from build123d import *

# Parameters (mm, degrees)
F0_W      = 200
F0_H      = 100
F0_W_2    = 196
F0_H_2    = 96
F1_DEPTH  = 40
F2_DEPTH  = 2
F3_W      = 62
F3_H      = 96
F4_DEPTH  = 25
F5_W      = 60
F5_H      = 96
F6_DEPTH  = 25
F8_DEPTH  = 25
F9_W      = 14
F9_H      = 10
F10_DEPTH = 5
F12_W     = 10
F12_H     = 10
F13_DEPTH = 5
F14_R     = 2
F15_W     = 20
F15_H     = 15
F16_DEPTH = 2
F17_W     = 15
F17_H     = 10
F18_DEPTH = 2
F19_W     = 86
F19_H     = 2
F20_DEPTH = 25
F21_W     = 25
F21_H     = 15
F22_DEPTH = 88
F23_W     = 40
F23_H     = 30
F24_DEPTH = 2
F25_W     = 20
F25_H     = 15
F26_DEPTH = 2


with BuildPart() as f1:
    # F0 (on Front) → F1 (new body)
    with BuildSketch(Plane.XZ):
        with Locations((-23.666499, -18.106852)):
            Rectangle(F0_W, F0_H)
        with Locations((-23.666499, -18.106852)):
            Rectangle(F0_W_2, F0_H_2, mode=Mode.SUBTRACT)
    extrude(amount=F1_DEPTH)

    # F0 (on Front) → F2 (join)
    with BuildSketch(Plane.XZ):
        with Locations((-23.666499, -18.106852)):
            Rectangle(F0_W_2, F0_H_2)
    extrude(amount=F2_DEPTH)

    # F3 (on face) → F4 (join)
    with BuildSketch(Plane.XZ.offset(2)):
        with Locations((-90.666499, -18.106852)):
            Rectangle(F3_W, F3_H)
    extrude(amount=F4_DEPTH)

    # F5 (on face) → F6 (cut)
    with BuildSketch(Plane.XZ.offset(27)):
        with Locations((-91.666499, -18.106852)):
            Rectangle(F5_W, F5_H)
    extrude(amount=-F6_DEPTH, mode=Mode.SUBTRACT)

    # F7 (on face) → F8 (join)
    with BuildSketch(Plane.XZ.offset(2)):
        Polygon((-11.666499, 29.893148), (-13.666499, 29.893148), (-13.666499, 14.893148), (-59.666499, 14.893148), (-59.666499, 12.893148), (-11.666499, 12.893148), align=None)
    extrude(amount=F8_DEPTH)

    # F9 (on face) → F10 (cut)
    with BuildSketch(Plane(origin=(0, 0, 12.893148), x_dir=(1, 0, 0), z_dir=(0, 0, -1))):
        with Locations((0.078483, 7)):
            Rectangle(F9_W, F9_H)
    extrude(amount=-F10_DEPTH, mode=Mode.SUBTRACT)

    # F12 (on face) → F13 (cut)
    with BuildSketch(Plane(origin=(-61.666499, 0, 0), x_dir=(0, -1, 0), z_dir=(-1, 0, 0))):
        with Locations((7, 21.893148)):
            Rectangle(F12_W, F12_H)
    extrude(amount=-F13_DEPTH, mode=Mode.SUBTRACT)

    # F14
    f14_edges = [f1.edges().sort_by_distance(p)[0] for p in [
        (76.333501, -20, -68.106852),
        (76.333501, -20, 31.893148),
        (-123.666499, -20, -68.106852),
        (-123.666499, -20, 31.893148),
    ]]
    fillet(f14_edges, radius=F14_R)

    # F15 (on face) → F16 (cut)
    with BuildSketch(Plane(origin=(0, 0, 12.893148), x_dir=(1, 0, 0), z_dir=(0, 0, -1))):
        with Locations((-35.666499, 9.5)):
            Rectangle(F15_W, F15_H)
    extrude(amount=-F16_DEPTH, mode=Mode.SUBTRACT)

    # F17 (on face) → F18 (cut)
    with BuildSketch(Plane.YZ.offset(-11.666499)):
        with Locations((-9.5, 21.393148)):
            Rectangle(F17_W, F17_H)
    extrude(amount=-F18_DEPTH, mode=Mode.SUBTRACT)

    # F19 (on face) → F20 (join)
    with BuildSketch(Plane.XZ.offset(2)):
        with Locations((31.333501, 13.893148)):
            Rectangle(F19_W, F19_H)
        with Locations((31.333501, 28.893148)):
            Rectangle(F19_W, F19_H)
    extrude(amount=F20_DEPTH)

    # F21 (on face) → F22 (cut)
    with BuildSketch(Plane(origin=(-13.666499, 0, 0), x_dir=(0, -1, 0), z_dir=(-1, 0, 0))):
        with Locations((14.5, 22.393148)):
            Rectangle(F21_W, F21_H)
    extrude(amount=-F22_DEPTH, mode=Mode.SUBTRACT)

    # F23 (on face) → F24 (cut)
    with BuildSketch(Plane(origin=(0, 0, -68.106852), x_dir=(1, 0, 0), z_dir=(0, 0, -1))):
        with Locations((54.333501, 15)):
            Rectangle(F23_W, F23_H)
    extrude(amount=-F24_DEPTH, mode=Mode.SUBTRACT)

    # F25 (on face) → F26 (cut)
    with BuildSketch(Plane(origin=(0, 0, 12.893148), x_dir=(1, 0, 0), z_dir=(0, 0, -1))):
        with Locations((64.333501, 9.5)):
            Rectangle(F25_W, F25_H)
    extrude(amount=-F26_DEPTH, mode=Mode.SUBTRACT)


solid = f1.part
For this review, take the finished solid that the model builds, in its own axes (mm). A direction names the side the tool comes from. Round coordinates to 2 decimals unless told otherwise and drop trailing zeros. Loops run counter-clockwise (first coordinate to the right, second up) from the corner with the lowest first, then second, coordinate; pieces in that order, holes last. Notation, with made-up numbers: (-34, 37.25) - (-20, 37.25) arc R29 cw to (-20, 62.25) - close; hole circle Ø3 at (37, 83). An arc over 180 degrees is marked (long way). One line per question, with ' | ' between items.
Q1. Take a section at B-B (x = -28.5). Give the boundary of the cut face in (y, z), and give its area (3 significant figures).
Taken from the geometry:
outline: (-40, -68.11) - (0, -68.11) - (0, 31.89) - (-40, 31.89) - (-40, 29.89) - (-2, 29.89) - (-2, -66.11) - (-40, -66.11) - close; (-27, 12.89) - (-17, 12.89) - (-17, 14.89) - (-27, 14.89) - close | area: 372 mm²
Q2. For pin 1 (1.5 mm diameter, centred on x = 41.5, y = -19.5, fed in from -Z); pin 2 (2 mm diameter, centred on x = 15.5, z = -34.5, fed in from -Y); pin 3 (0.6 mm diameter, centred on y = -18.5, z = -67.5, fed in from +X), all flat-tipped, find the tip position at first contact; note any pin that passes through.
Taken from the geometry:
pin 1: stops at z = 12.89 | pin 2: stops at y = -2 | pin 3: stops at x = 76.01
Q3. Take a section at D-D (x = 15.5). Give the boundary of the cut face in (y, z), and give its area (3 significant figures).
Taken from the geometry:
outline: (-40, -68.11) - (0, -68.11) - (0, 31.89) - (-40, 31.89) - (-40, 29.89) - (-2, 29.89) - (-2, 14.89) - (-27, 14.89) - (-27, 12.89) - (-2, 12.89) - (-2, -66.11) - (-40, -66.11) - close | area: 402 mm²
Q4. For line 1 along X through (y, z) = (-5.5, -26.5); line 2 along Z through (x, y) = (4, -8); line 3 along Z through (x, y) = (-95.5, -33.5), list the stretches that pass through material, from the lowest coordinate up. Write a range as [from, to].
Taken from the geometry:
line 1: x = [-123.67, -121.67], [-61.67, -59.67], [74.33, 76.33] | line 2: z = [-68.11, -66.11], [12.89, 14.89], [29.89, 31.89] | line 3: z = [-68.11, -66.11], [29.89, 31.89]
Q5. Take a section at A-A (y = -37). Give the boundary of the cut face in (x, z), and give its area (3 significant figures).
Taken from the geometry:
outline: (-123.67, -66.11) arc R2 ccw to (-121.67, -68.11) - (74.33, -68.11) arc R2 ccw to (76.33, -66.11) - (76.33, 29.89) arc R2 ccw to (74.33, 31.89) - (-121.67, 31.89) arc R2 ccw to (-123.67, 29.89) - close; hole (-121.67, -66.11) - (74.33, -66.11) - (74.33, 29.89) - (-121.67, 29.89) - close | area: 1,180 mm²
Q6. The part is to be moulded in two halves that separate along X. For faces 3 (the flat face through (-123.666, -20, -19)), 4 (the flat face through (6, -27, 14)), 5 (the flat face through (-25, 0, -17)), say which applies: released by +X, released by -X, zero draft, split by the parting line, or undercut.
Taken from the geometry:
face 3: released by -X | face 4: undercut | face 5: zero draft
Q7. Tool access review of faces 1 (the flat face through (8, -14, 14.893)), 2 (the flat face through (76.334, -20, -19)): name each direction out of +Z, -Z, +X, -X, +Y, -Y from which nothing blocks a thin tool from reaching the whole face with its end or side.
Taken from the geometry:
face 1: -Y | face 2: +Z, -Z, +X, +Y, -Y
Q8. Take a section at C-C (z = 20.5). Give the boundary of the cut face in (x, y).
Taken from the geometry:
outline: (-123.67, -40) - (-121.67, -40) - (-121.67, -2) - (74.33, -2) - (74.33, -40) - (76.33, -40) - (76.33, 0) - (-123.67, 0) - close; (-61.67, -27) - (-59.67, -27) - (-59.67, -12) - (-61.67, -12) - close
